from build123d import *

# Parameters (mm, degrees)
BOSS_EXTRUDE1_DEPTH = 1.499997
FILLET1_R           = 2.0193


with BuildPart() as part:
    # Sketch1 → Boss-Extrude1 (new, symmetric)
    with BuildSketch(Plane.XY):
        with BuildLine():
            ThreePointArc((-13.645493623, 4.234756195), (-14.2875, 0), (-13.645493623, -4.234756195))
            ThreePointArc((-13.645493623, -4.234756195), (-15.122968614, -8.73125), (-10.490153255, -9.699966028))
            ThreePointArc((-10.490153255, -9.699966028), (-7.14375, -12.373337957), (-3.155340368, -13.934722222))
            ThreePointArc((-3.155340368, -13.934722222), (0, -17.4625), (3.155340368, -13.934722222))
            ThreePointArc((3.155340368, -13.934722222), (7.14375, -12.373337957), (10.490153255, -9.699966028))
            ThreePointArc((10.490153255, -9.699966028), (15.122968614, -8.73125), (13.645493623, -4.234756195))
            ThreePointArc((13.645493623, -4.234756195), (14.2875, 0), (13.645493623, 4.234756195))
            ThreePointArc((13.645493623, 4.234756195), (15.122968614, 8.73125), (10.490153255, 9.699966028))
            ThreePointArc((10.490153255, 9.699966028), (7.14375, 12.373337957), (3.155340368, 13.934722222))
            ThreePointArc((3.155340368, 13.934722222), (0, 17.4625), (-3.155340368, 13.934722222))
            ThreePointArc((-3.155340368, 13.934722222), (-7.14375, 12.373337957), (-10.490153255, 9.699966028))
            ThreePointArc((-10.490153255, 9.699966028), (-15.122968614, 8.73125), (-13.645493623, 4.234756195))
        make_face()
        Polygon((0, 7.478995387), (-6.477, 3.739497694), (-6.477, -3.739497694), (0, -7.478995387), (6.477, -3.739497694), (6.477, 3.739497694), align=None, mode=Mode.SUBTRACT)
    extrude(amount=BOSS_EXTRUDE1_DEPTH, both=True)

    # Fillet1
    fillet1_edges = [part.edges().sort_by_distance(p)[0] for p in [
        (10.490153255, 9.699966028, 0),
        (13.645493623, 4.234756195, 0),
        (13.645493623, -4.234756195, 0),
        (10.490153255, -9.699966028, 0),
        (3.155340368, -13.934722222, 0),
        (-3.155340368, -13.934722222, 0),
        (-10.490153255, -9.699966028, 0),
        (-13.645493623, -4.234756195, 0),
        (-13.645493623, 4.234756195, 0),
        (-10.490153255, 9.699966028, 0),
        (-3.155340368, 13.934722222, 0),
        (3.155340368, 13.934722222, 0),
    ]]
    fillet(fillet1_edges, radius=FILLET1_R)


solid = part.part
Can you work these out from the model? Positions are in its coordinate system, mm. A direction names the side the tool comes from. Coordinates: 2 decimals unless noted, no trailing zeros. Order: outer loops, then holes, each group sorted by start corner. A loop starts at its lowest first (then second) coordinate and runs counter-clockwise, first axis right, second up. Notation, with made-up numbers: (50.25, -26) - (71.25, -26) arc R5 ccw to (71.25, -22) - close; hole circle Ø3 at (60.5, 47.5). An arc over 180 degrees is marked (long way). Answer as a JSON object with one key per item and string values. Group by question number.
Q1. Imagine slicing it at C-C (y = 12). Please give me the cut outline in (x, z), and give its area (3 significant figures).
Q2. We'd pull the mould along Y, two halves only. Please class faces 3 (the face through (-15.15, -8.68, 0.02)), 4 (the face through (0.06, 17.46, 0.02)), 5 (the face through (7, 0, -1.5)), 6 (the face through (-7.18, -12.352, 0.021)): +Y half, -Y half, draft (parallel to the pull), parting line (faces both ways), or undercut.
Q3. Will this pin go through, and if not, where does the flat tip stop? P1, Ø1, axis at x = -12.5, z = -0.5, coming from the +Y side.
Q4. I need wall thicknesses on line 1 (X direction, y = 3.5, z = -1.25); line 2 (X direction, y = 0, z = -0.45); line 3 (X direction, y = 15, z = -0.7). Which ranges of each line are inside material? Lowest first, please. Write a range as from..to.
Q5. On a 3-axis mill with a long thin cutter (end or side, diameter ignored), from which of +Z, -Z, +X, -X, +Y, -Y can I reach the whole of each face in a straight line? I mean faces 1 (the face through (3.284, 5.583, 0.021)), 2 (the face through (-14.287, 0.042, 0.021)). Say none if no direction works.
Q6. Imagine slicing it at B-B (x = -5). Please give me the cut outline in (y, z).
Q7. Imagine slicing it at A-A (y = -7). Please give me the cut outline in (x, z), and give its area (3 significant figures).
Q8. Imagine slicing it at D-D (x = 8). Please give me the cut outline in (y, z), and give its area (3 significant figures).
Determined:
{
 "1": {"outline": "(-7.75, -1.5) - (7.75, -1.5) - (7.75, 1.5) - (-7.75, 1.5) - close", "area": "46.5 mm2"},
 "2": {"face 3": "undercut", "face 4": "+Y half", "face 5": "draft", "face 6": "-Y half"},
 "3": {"P1": "stops at y = 10.32"},
 "4": {"line 1": "x = -13.94..-6.48, 6.48..13.94", "line 2": "x = -14.29..-6.48, 6.48..14.29", "line 3": "x = -3.09..3.09"},
 "5": {"face 1": "+Z, -Z", "face 2": "+Z, -Z, -X"},
 "6": {"outline": "(-13.38, -1.5) - (-4.59, -1.5) - (-4.59, 1.5) - (-13.38, 1.5) - close; (4.59, -1.5) - (13.38, -1.5) - (13.38, 1.5) - (4.59, 1.5) - close"},
 "7": {"outline": "(-15.55, -1.5) - (-0.83, -1.5) - (-0.83, 1.5) - (-15.55, 1.5) - close; (0.83, -1.5) - (15.55, -1.5) - (15.55, 1.5) - (0.83, 1.5) - close", "area": "88.3 mm2"},
 "8": {"outline": "(-11.84, -1.5) - (11.84, -1.5) - (11.84, 1.5) - (-11.84, 1.5) - close", "area": "71.0 mm2"}
}
